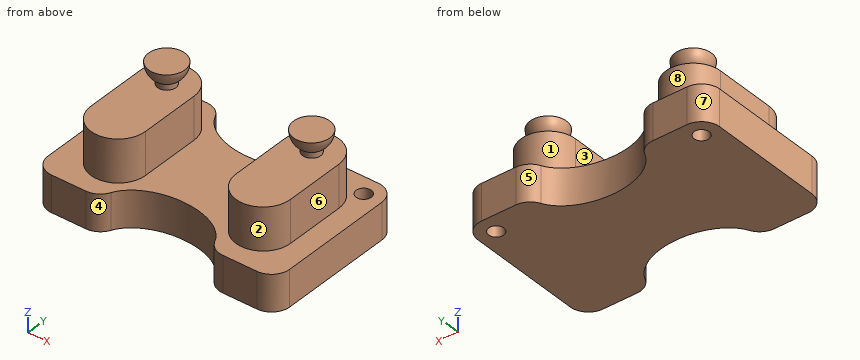
from build123d import *

# Parameters (mm, degrees)
SKIZZE1_W                       = 40
SKIZZE1_H                       = 25
AUFSATZ_LINEAR_AUSTRAGEN1_DEPTH = 6
AUFSATZ_LINEAR_AUSTRAGEN2_DEPTH = 7
SKIZZE3_R                       = 1.5
AUFSATZ_LINEAR_AUSTRAGEN3_DEPTH = 3.5
ROTATION1_ANGLE                 = 180
VERRUNDUNG1_R                   = 3
SKIZZE6_RX                      = 9
SKIZZE6_RY                      = 6
SCHNITT_LINEAR_AUSTRAGEN7_DEPTH = 6
VERRUNDUNG2_START               = -1
VERRUNDUNG2_DEPTH               = 8
VERRUNDUNG3_START               = -1
VERRUNDUNG3_DEPTH               = 8
SKIZZE7_R                       = 1.25
SCHNITT_LINEAR_AUSTRAGEN8_DEPTH = 6


with BuildPart() as part:
    # Skizze1 → Aufsatz-Linear austragen1 (new body)
    with BuildSketch(Plane.XY):
        with Locations((20, 12.5)):
            Rectangle(SKIZZE1_W, SKIZZE1_H)
    extrude(amount=AUFSATZ_LINEAR_AUSTRAGEN1_DEPTH)

    # Skizze2 → Aufsatz-Linear austragen2 (add)
    with BuildSketch(Plane.XY.offset(6)):
        with BuildLine():
            Line((12.5, 17.5), (12.5, 7.5))
            ThreePointArc((12.5, 7.5), (8, 3), (3.5, 7.5))
            Line((3.5, 7.5), (3.5, 17.5))
            ThreePointArc((3.5, 17.5), (8, 22), (12.5, 17.5))
        make_face()
    aufsatz_linear_austragen2 = extrude(amount=AUFSATZ_LINEAR_AUSTRAGEN2_DEPTH)

    # Spiegeln1: Aufsatz-Linear austragen2 across plane
    add(aufsatz_linear_austragen2.mirror(Plane.ZY.offset(-20)))

    # Skizze3 → Aufsatz-Linear austragen3 (add)
    with BuildSketch(Plane.XY.offset(13)):
        with Locations((8, 17.5)):
            Circle(SKIZZE3_R)
    aufsatz_linear_austragen3 = extrude(amount=AUFSATZ_LINEAR_AUSTRAGEN3_DEPTH)

    # Spiegeln2: Aufsatz-Linear austragen3 across plane
    add(aufsatz_linear_austragen3.mirror(Plane.ZY.offset(-20)))

    # Skizze4 → Rotation1 (revolve)
    with BuildSketch(Plane.XY.offset(16.5)):
        with BuildLine():
            Line((5, 17.5), (11, 17.5))
            ThreePointArc((11, 17.5), (8, 14.5), (5, 17.5))
        make_face()
    rotation1 = revolve(axis=Axis((5, 17.5, 16.5), (1, 0, 0)), revolution_arc=ROTATION1_ANGLE)

    # Spiegeln3: Rotation1 across plane
    add(rotation1.mirror(Plane.ZY.offset(-20)))

    # Verrundung1
    verrundung1_edges = [part.edges().sort_by_distance(p)[0] for p in [
        (0, 25, 3),
        (40, 25, 3),
        (40, 0, 3),
        (0, 0, 3),
    ]]
    fillet(verrundung1_edges, radius=VERRUNDUNG1_R)

    # Skizze6 → Schnitt-Linear austragen7 (cut)
    with BuildSketch(Plane.XY.offset(6)):
        with Locations(Location((20, 0), (0, 0, 180))):
            Ellipse(SKIZZE6_RX, SKIZZE6_RY)
    schnitt_linear_austragen7 = extrude(amount=-SCHNITT_LINEAR_AUSTRAGEN7_DEPTH, mode=Mode.SUBTRACT)

    # Verrundung2: read off the stored shape, not the designer's step
    # Verrundung2 outline → Verrundung2 (cut)
    with BuildSketch(Plane.XY.offset(VERRUNDUNG2_START)):
        with BuildLine():
            add(Edge.make_bspline(
                [(11.391923436, 1.751319232), (11, 0.89515019), (11, 0)],
                knots=[5.971053557, 5.971053557, 5.971053557, 6.283185307, 6.283185307, 6.283185307], degree=2, weights=[0.906728811, 0.94179941, 1]))
            ThreePointArc((11.391923436, 1.751319232), (10.28493687, 0.475515666), (8.664141124, 0))
            Line((8.664141124, 0), (11, 0))
        make_face()
        with BuildLine():
            ThreePointArc((31.335858876, 0), (29.71506313, 0.475515666), (28.608076564, 1.751319232))
            add(Edge.make_bspline(
                [(29, 0), (29, 0.89515019), (28.608076564, 1.751319232)],
                knots=[3.141592654, 3.141592654, 3.141592654, 3.453724403, 3.453724403, 3.453724403], degree=2, weights=[1, 0.94179941, 0.906728811]))
            Line((29, 0), (31.335858876, 0))
        make_face()
    extrude(amount=VERRUNDUNG2_DEPTH, mode=Mode.SUBTRACT)

    # Spiegeln5: Schnitt-Linear austragen7 across plane
    add(schnitt_linear_austragen7.mirror(Plane.ZX.offset(12.5)), mode=Mode.SUBTRACT)

    # Verrundung3: read off the stored shape, not the designer's step
    # Verrundung3 outline → Verrundung3 (cut)
    with BuildSketch(Plane.XY.offset(VERRUNDUNG3_START)):
        with BuildLine():
            ThreePointArc((8.664141124, 25), (10.28493687, 24.524484334), (11.391923436, 23.248680768))
            add(Edge.make_bspline(
                [(11.391923436, 23.248680768), (11, 24.10484981), (11, 25)],
                knots=[5.971053557, 5.971053557, 5.971053557, 6.283185307, 6.283185307, 6.283185307], degree=2, weights=[0.906728811, 0.94179941, 1]))
            Line((11, 25), (8.664141124, 25))
        make_face()
        with BuildLine():
            ThreePointArc((28.608076564, 23.248680768), (29.71506313, 24.524484334), (31.335858876, 25))
            Line((31.335858876, 25), (29, 25))
            add(Edge.make_bspline(
                [(29, 25), (29, 24.10484981), (28.608076564, 23.248680768)],
                knots=[3.141592654, 3.141592654, 3.141592654, 3.453724403, 3.453724403, 3.453724403], degree=2, weights=[1, 0.94179941, 0.906728811]))
        make_face()
    extrude(amount=VERRUNDUNG3_DEPTH, mode=Mode.SUBTRACT)

    # Skizze7 → Schnitt-Linear austragen8 (cut)
    with BuildSketch(Plane.XY.offset(6)):
        with Locations((3, 22)):
            Circle(SKIZZE7_R)
    schnitt_linear_austragen8 = extrude(amount=-SCHNITT_LINEAR_AUSTRAGEN8_DEPTH, mode=Mode.SUBTRACT)

    # Spiegeln6: Schnitt-Linear austragen8 across plane
    add(schnitt_linear_austragen8.mirror(Plane.ZY.offset(-20)), mode=Mode.SUBTRACT)


solid = part.part
Work out the finished part from the listing and answer in its coordinate system (mm). Face numbers are marked on the shaded views. A direction names the side the tool comes from. Round coordinates to 2 decimals unless told otherwise and drop trailing zeros. Loops run counter-clockwise (first coordinate to the right, second up) from the corner with the lowest first, then second, coordinate; pieces in that order, holes last. Notation, with made-up numbers: (43.5, 29.25) - (52.5, 29.25) arc R22 cw to (52.5, 62.25) - close; hole circle Ø3 at (58.25, -9.5). An arc over 180 degrees is marked (long way). One line per item, written item: value.
Q1. Straight lines are drawn through the part: probe 1 along Y at (x, z) = (3, 3); probe 2 along X at (y, z) = (13, 9.25); probe 3 along Z at (x, y) = (16.5, 9.75). For each, find the intervals that lie inside material, in ascending order.
Check values:
probe 1: 0 to 20.75, 23.25 to 25
probe 2: 3.5 to 12.5, 27.5 to 36.5
probe 3: 0 to 6
Q2. The mould has two halves that part along X. Classify the marked faces 5, 6, 7 and 8: +X half, -X half, draft (parallel to the pull), parting line (faces both ways), or undercut.
Check values:
face 5: undercut
face 6: +X half
face 7: -X half
face 8: undercut
Q3. Find section C-C on y = 12.25. Give the vertices of the cut face in (x, z), and give its area (3 significant figures).
Check values:
outline: (0, 0) - (40, 0) - (40, 6) - (36.5, 6) - (36.5, 13) - (27.5, 13) - (27.5, 6) - (12.5, 6) - (12.5, 13) - (3.5, 13) - (3.5, 6) - (0, 6) - close
area: 366 mm2
Q4. Find section A-A on z = 10.5. Give the vertices of the cut face in (x, y), and give its area (3 significant figures).
Check values:
outline: (3.5, 7.5) arc R4.5 ccw to (12.5, 7.5) - (12.5, 17.5) arc R4.5 ccw to (3.5, 17.5) - close; (27.5, 7.5) arc R4.5 ccw to (36.5, 7.5) - (36.5, 17.5) arc R4.5 ccw to (27.5, 17.5) - close
area: 307 mm2
Q5. Find section D-D on x = 8. Give the vertices of the cut face in (y, z).
Check values:
outline: (0, 0) - (25, 0) - (25, 6) - (22, 6) - (22, 13) - (19, 13) - (19, 13.9) arc R3 ccw to (20.5, 16.5) - (14.5, 16.5) arc R3 ccw to (16, 13.9) - (16, 13) - (3, 13) - (3, 6) - (0, 6) - close
Q6. For the marked faces 1, 2, 3 and 4, determine the directions among +Z, -Z, +X, -X, +Y, -Y from which every point of the face is accessible in a straight line to the end or side of a thin tool.
Check values:
face 1: +Z, +Y
face 2: +Z, -Y
face 3: +Z, +Y, -Y
face 4: +Z, -Z, -Y
Q7. Find section B-B on x = 30. Give the vertices of the cut face in (y, z).
Check values:
outline: (0.31, 0) - (24.69, 0) - (24.69, 6) - (21.53, 6) - (21.53, 13) - (3.47, 13) - (3.47, 6) - (0.31, 6) - close; (15.26, 16.5) arc R2.24 ccw to (19.74, 16.5) - close
Q8. Each of these flat-tipped pins is pushed along its axis until it touches: pin 1 Ø3 at (x, y) = (37, 22) entering from -Z; pin 2 Ø2 at (y, z) = (11, 11) entering from +X; pin 3 Ø12.5 at (x, y) = (22, 9) entering from +Z; pin 4 Ø4 at (y, z) = (3.5, 12.5) entering from -X. Where does it stop, or does it pass through?
Check values:
pin 1: z = 0
pin 2: x = 36.5
pin 3: z = 13
pin 4: x = 3.97
